For this review, take the finished solid that the model builds, in its own axes (mm). Round coordinates to 2 decimals unless told otherwise and drop trailing zeros. Write each loop counter-clockwise with the first axis right and the second up, starting at its lowest first coordinate (ties: lowest second). Pieces come first, ordered by that corner, then holes.
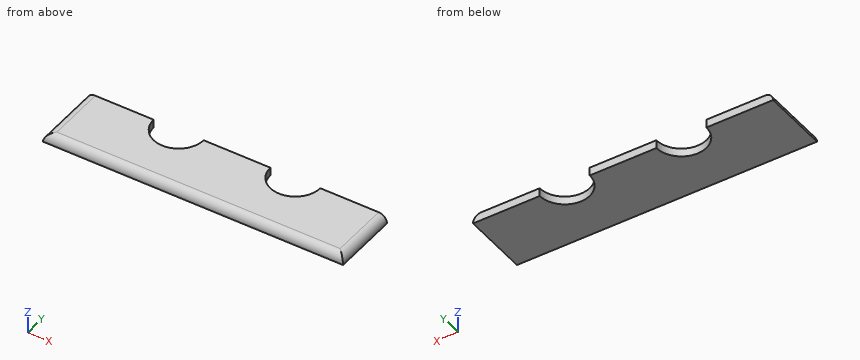
from build123d import *

# Parameters (mm, degrees)
F1_DEPTH = 5
F2_R     = 4.99999


# Not quite as in the source:
# - a fillet or chamfer is up to 0.001 mm smaller than in the source, because OpenCascade refuses the exact size


with BuildPart() as f1:
    # F0 (on Top) → F1 (new body)
    with BuildSketch(Plane.XY):
        with BuildLine():
            Line((20, 0), (0, 0))
            Line((0, 0), (-20, 0))
            ThreePointArc((-20, 0), (-35, -15), (-50, 0))
            Line((-50, 0), (-90, 0))
            Line((-90, 0), (-90, -40))
            Line((-90, -40), (0, -40))
            Line((0, -40), (90, -40))
            Line((90, -40), (90, 0))
            Line((90, 0), (50, 0))
            ThreePointArc((50, 0), (35, -15), (20, 0))
        make_face()
    extrude(amount=F1_DEPTH)

    # F2 (radius 5 in the source; OpenCascade refuses exactly that, so slightly less here)
    f2_edges = [f1.edges().sort_by_distance(p)[0] for p in [
        (0, -40, 5),
        (-90, -20, 5),
        (90, -20, 5),
    ]]
    fillet(f2_edges, radius=F2_R)


solid = f1.part
(1) We need section A-A, the plane y = -12. State how many separate pieces and enclosed holes the cut face has, and give its area (3 significant figures).
Geometry check:
separate pieces: 3
enclosed holes: 0
area: 709 mm2
(2) We need section C-C, the plane z = 3.85. Give the boundary of the cut face in (x, y), and give its area (3 significant figures).
Geometry check:
outline: (-88.19, -38.19) - (88.19, -38.19) - (88.19, 0) - (50, 0) arc R15 cw to (20, 0) - (-20, 0) arc R15 cw to (-50, 0) - (-88.19, 0) - close
area: 6,030 mm2
(3) For pin 1 Ø1.5 at (y, z) = (-18.5, 3.5) entering from -X, flat-tipped, find the tip position at first contact; note if it passes through.
Geometry check:
pin 1: stops at x = -89.18
(4) For line 1 along X through (y, z) = (-13, 1.4); line 2 along X through (y, z) = (-6.5, 4.6); line 3 along X through (y, z) = (-27.5, 0.6), list the stretches that pass through material, from the lowest coordinate up.
Geometry check:
line 1: x = -89.8 to -42.48, -27.52 to 27.52, 42.48 to 89.8
line 2: x = -86.96 to -48.52, -21.48 to 21.48, 48.52 to 86.96
line 3: x = -89.96 to 89.96
